The model under review builds one solid part; all positions refer to its coordinate system, in mm. Face numbers are marked on the shaded views. A direction names the side the tool comes from. Coordinates: 2 decimals unless noted, no trailing zeros. Write each loop counter-clockwise with the first axis right and the second up, starting at its lowest first coordinate (ties: lowest second). Pieces come first, ordered by that corner, then holes. Notation, with made-up numbers: M 68.25,53.5 L 125.25,53.5 A18 cw 125.25,85.5 Z; hole C 70,71 d2. An arc over 180 degrees is marked long. Answer as a JSON object with one key per item and string values.
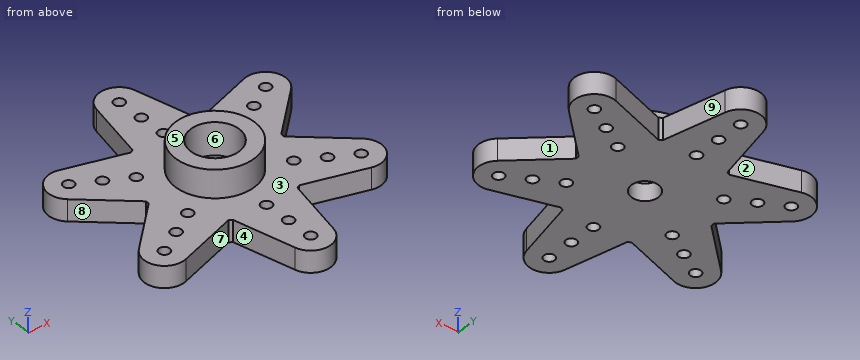
```python
from build123d import *

# Parameters (mm, degrees)
SKIZZE1_R                       = 1.5
SKIZZE1_R_2                     = 0.6
AUFSATZ_LINEAR_AUSTRAGEN1_DEPTH = 2.4
SKIZZE2_R                       = 4.4
SKIZZE2_R_2                     = 1.5
AUFSATZ_LINEAR_AUSTRAGEN2_DEPTH = 3.1
SKIZZE4_R                       = 2.7
SCHNITT_LINEAR_AUSTRAGEN1_DEPTH = 3.6


with BuildPart() as part:
    # Skizze1 → Aufsatz-Linear austragen1 (new body)
    with BuildSketch(Plane.XY):
        with BuildLine():
            Line((-3.7, 6.809735678), (-2.195055787, 13.494196411))
            ThreePointArc((-2.195055787, 13.494196411), (0, 15.25), (2.195055787, 13.494196411))
            Line((2.195055787, 13.494196411), (3.7, 6.809735678))
            Line((3.7, 6.809735678), (4.04740409, 6.609161833))
            Line((4.04740409, 6.609161833), (10.588789002, 8.64807228))
            ThreePointArc((10.588789002, 8.64807228), (13.206887408, 7.625), (12.783844789, 4.846124131))
            Line((12.783844789, 4.846124131), (7.74740409, 0.200573845))
            Line((7.74740409, 0.200573845), (7.74740409, -0.200573845))
            Line((7.74740409, -0.200573845), (12.783844789, -4.846124131))
            ThreePointArc((12.783844789, -4.846124131), (13.206887408, -7.625), (10.588789002, -8.64807228))
            Line((10.588789002, -8.64807228), (4.04740409, -6.609161833))
            Line((4.04740409, -6.609161833), (3.7, -6.809735678))
            Line((3.7, -6.809735678), (2.195055787, -13.494196411))
            ThreePointArc((2.195055787, -13.494196411), (0, -15.25), (-2.195055787, -13.494196411))
            Line((-2.195055787, -13.494196411), (-3.7, -6.809735678))
            Line((-3.7, -6.809735678), (-4.04740409, -6.609161833))
            Line((-4.04740409, -6.609161833), (-10.588789002, -8.64807228))
            ThreePointArc((-10.588789002, -8.64807228), (-13.206887408, -7.625), (-12.783844789, -4.846124131))
            Line((-12.783844789, -4.846124131), (-7.74740409, -0.200573845))
            Line((-7.74740409, -0.200573845), (-7.74740409, 0.200573845))
            Line((-7.74740409, 0.200573845), (-12.783844789, 4.846124131))
            ThreePointArc((-12.783844789, 4.846124131), (-13.206887408, 7.625), (-10.588789002, 8.64807228))
            Line((-10.588789002, 8.64807228), (-4.04740409, 6.609161833))
            Line((-4.04740409, 6.609161833), (-3.7, 6.809735678))
        make_face()
        Circle(SKIZZE1_R, mode=Mode.SUBTRACT)
        with Locations((0, 13)):
            Circle(SKIZZE1_R_2, mode=Mode.SUBTRACT)
        with Locations((0, 10)):
            Circle(SKIZZE1_R_2, mode=Mode.SUBTRACT)
        with Locations((0, 7)):
            Circle(SKIZZE1_R_2, mode=Mode.SUBTRACT)
        with Locations((6.062177826, 3.5)):
            Circle(SKIZZE1_R_2, mode=Mode.SUBTRACT)
        with Locations((8.660254038, 5)):
            Circle(SKIZZE1_R_2, mode=Mode.SUBTRACT)
        with Locations((11.258330249, 6.5)):
            Circle(SKIZZE1_R_2, mode=Mode.SUBTRACT)
        with Locations((6.062177826, -3.5)):
            Circle(SKIZZE1_R_2, mode=Mode.SUBTRACT)
        with Locations((8.660254038, -5)):
            Circle(SKIZZE1_R_2, mode=Mode.SUBTRACT)
        with Locations((11.258330249, -6.5)):
            Circle(SKIZZE1_R_2, mode=Mode.SUBTRACT)
        with Locations((0, -7)):
            Circle(SKIZZE1_R_2, mode=Mode.SUBTRACT)
        with Locations((0, -10)):
            Circle(SKIZZE1_R_2, mode=Mode.SUBTRACT)
        with Locations((0, -13)):
            Circle(SKIZZE1_R_2, mode=Mode.SUBTRACT)
        with Locations((-6.062177826, -3.5)):
            Circle(SKIZZE1_R_2, mode=Mode.SUBTRACT)
        with Locations((-8.660254038, -5)):
            Circle(SKIZZE1_R_2, mode=Mode.SUBTRACT)
        with Locations((-11.258330249, -6.5)):
            Circle(SKIZZE1_R_2, mode=Mode.SUBTRACT)
        with Locations((-6.062177826, 3.5)):
            Circle(SKIZZE1_R_2, mode=Mode.SUBTRACT)
        with Locations((-8.660254038, 5)):
            Circle(SKIZZE1_R_2, mode=Mode.SUBTRACT)
        with Locations((-11.258330249, 6.5)):
            Circle(SKIZZE1_R_2, mode=Mode.SUBTRACT)
    extrude(amount=AUFSATZ_LINEAR_AUSTRAGEN1_DEPTH)

    # Skizze2 → Aufsatz-Linear austragen2 (add)
    with BuildSketch(Plane.XY.offset(2.4)):
        with Locations(Location((0, 0, 0), (0, 0, 180))):
            Circle(SKIZZE2_R)
        Circle(SKIZZE2_R_2, mode=Mode.SUBTRACT)
    extrude(amount=AUFSATZ_LINEAR_AUSTRAGEN2_DEPTH)

    # Skizze4 → Schnitt-Linear austragen1 (cut)
    with BuildSketch(Plane.XY.offset(5.5)):
        Circle(SKIZZE4_R)
    extrude(amount=-SCHNITT_LINEAR_AUSTRAGEN1_DEPTH, mode=Mode.SUBTRACT)


solid = part.part
```
(1) Draft analysis for pull direction Y (two halves, no side actions). For the marked faces 1, 2, 3 and 4, state which applies: released by +Y, released by -Y, zero draft, split by the parting line, or undercut.
Results list:
{"face 1": "undercut", "face 2": "released by +Y", "face 3": "zero draft", "face 4": "released by -Y"}
(2) Add section D-D on y = 10. Give the boundary of the cut face in (x, z), and give its area (3 significant figures).
Results list:
{"outline": "M -2.98,0 L -0.6,0 L -0.6,2.4 L -2.98,2.4 Z; M 0.6,0 L 2.98,0 L 2.98,2.4 L 0.6,2.4 Z", "area": "11.4 mm²"}
(3) For the marked faces 5, 6, 7, 8 and 9, list the 3-axis set-ups (+Z, -Z, +X, -X, +Y, -Y) from which the entire face can be reached by the end or side of a thin tool; tool diameter is ignored.
Results list:
{"face 5": "+Z, +X, -X, +Y, -Y", "face 6": "+Z", "face 7": "+Z, -Z, -Y", "face 8": "+Z, -Z, -X", "face 9": "+Z, -Z, +Y"}
(4) Add section B-B on y = 3.5. Give the boundary of the cut face in (x, z), and give its area (3 significant figures).
Results list:
{"outline": "M -11.32,0 L -6.66,0 L -6.66,2.4 L -11.32,2.4 Z; M -5.46,0 L 5.46,0 L 5.46,2.4 L 2.67,2.4 L 2.67,5.5 L -2.67,5.5 L -2.67,2.4 L -5.46,2.4 Z; M 6.66,0 L 11.32,0 L 11.32,2.4 L 6.66,2.4 Z", "area": "65.1 mm²"}
(5) Add section A-A on x = -1. Give the boundary of the cut face in (y, z).
Results list:
{"outline": "M -15.02,0 L -1.12,0 L -1.12,1.9 L -2.51,1.9 L -2.51,5.5 L -4.28,5.5 L -4.28,2.4 L -15.02,2.4 Z; M 1.12,0 L 15.02,0 L 15.02,2.4 L 4.28,2.4 L 4.28,5.5 L 2.51,5.5 L 2.51,1.9 L 1.12,1.9 Z"}
(6) Wall thickness on line 1 along Y through (x, z) = (-11.75, 0.3); line 2 along X through (y, z) = (-6, 2); line 3 along X through (y, z) = (3, 1.1): over which ranges is each line inside the solid? List them lowest first. Write a range as from..to.
Results list:
{"line 1": "-8.7..-6.84, -6.16..-3.89, 3.89..6.16, 6.84..8.7", "line 2": "-13.45..-11.59, -10.93..10.93, 11.59..13.45", "line 3": "-10.78..-6.39, -5.73..5.73, 6.39..10.78"}
(7) For pin 1 Ø1 at (x, z) = (-8, 2.5) entering from +Y; pin 2 Ø1 at (y, z) = (1, 2.5) entering from -X; pin 3 Ø0.7 at (x, y) = (-11.26, -6.5) entering from -Z; pin 4 Ø1.9 at (x, y) = (8.66, 5) entering from +Z, all flat-tipped, find the tip position at first contact; note any pin that passes through.
Results list:
{"pin 1": "y = 7.99", "pin 2": "x = -9.15", "pin 3": "through", "pin 4": "z = 2.4"}
(8) Add section C-C on z = 2.9. Give the boundary of the cut face in (x, y), and give its area (3 significant figures).
Results list:
{"outline": "C 0,0 d8.8; hole C 0,0 d5.4", "area": "37.9 mm²"}
